Model file for the job. Use its own axes, mm. A direction names the side the tool comes from. Coordinates: 2 decimals unless noted, no trailing zeros. Write each loop counter-clockwise with the first axis right and the second up, starting at its lowest first coordinate (ties: lowest second). Pieces come first, ordered by that corner, then holes. Notation, with made-up numbers: M -2,7.25 L 23,7.25 A3 cw 23,12.25 Z; hole C 69,-2.75 d9. An arc over 180 degrees is marked long. Put each result on its own line as item: value. Start each with the question number.
Q1. Cut at B-B (z = 59.5). Write the cut outline in (x, y).
Q2. Drop flat-ended pins along their axis: pin 1 (4 mm diameter, centred on x = 11.5, z = 10, fed in from -Y); pin 2 (6 mm diameter, centred on x = 1.5, z = 39, fed in from +Y); pin 3 (1.5 mm diameter, centred on x = 10, y = -10.5, fed in from -Z); pin 4 (4 mm diameter, centred on x = -12, z = 88, fed in from -Y). Give the stop position or say it passes through.
Q3. Which spindle directions (+Z, -Z, +X, -X, +Y, -Y) get a long thin tool onto all of the face, cutting with end or side? Do faces 4 (the flat face through (-11.5, 5.9, 100)), 5 (the flat face through (0, 20, 33)), 6 (the cylindrical face through (11.923, -3.755, -32.955)). Say none if no direction does.
Q4. Cut at D-D (x = 21). Write the cut outline in (y, z), then the cut area to 3 significant figures.
Q5. Pull direction Z, two halves, no side cores. Call faces 1 (the cylindrical face through (-20, -15, 49)), 2 (the flat face through (0, 22, 70)), 3 (the flat face through (0, 0, 165)): pulls with the +Z half, pulls with the -Z half, needs draft (parallel to the pull), parting line crosses it, or undercut.
Q6. Cut at A-A (y = 0). Write the cut outline in (x, z).
Q7. Cut at C-C (z = 6). Write the cut outline in (x, y), then the cut area to 3 significant figures.
Q8. Drill centre lines: line 1 along Z through (x, y) = (19.5, -15.5); line 2 along Z through (x, y) = (-0.5, -22); line 3 along Z through (x, y) = (-11.5, -5). Where is each one in solid material? Low to high.
```python
from build123d import *

# Parameters (mm, degrees)
IZIM1_R                     = 25
Y_KSEKLIK_EKSTR_ZYON1_DEPTH = 100
IZIM2_R                     = 12.5
Y_KSEKLIK_EKSTR_ZYON2_DEPTH = 65
Y_KSEKLIK_EKSTR_ZYON3_START = 65
IZIM3_R                     = 12.5
Y_KSEKLIK_EKSTR_ZYON3_DEPTH = 65
KES_EKSTR_ZYON1_DEPTH       = 65
KES_EKSTR_ZYON1_DEPTH_BACK  = 65
KES_EKSTR_ZYON2_START       = 20
IZIM5_W                     = 40
IZIM5_H                     = 40
KES_EKSTR_ZYON2_DEPTH       = 10


with BuildPart() as part:
    # izim1 → Y_kseklik-Ekstr_zyon1 (new body)
    with BuildSketch(Plane.XY):
        Circle(IZIM1_R)
    extrude(amount=Y_KSEKLIK_EKSTR_ZYON1_DEPTH)

    # izim2 → Y_kseklik-Ekstr_zyon2 (add)
    with BuildSketch(Plane.XY.offset(100)):
        Circle(IZIM2_R)
    extrude(amount=Y_KSEKLIK_EKSTR_ZYON2_DEPTH)

    # izim3 → Y_kseklik-Ekstr_zyon3 (add)
    with BuildSketch(Plane(origin=(0, 0, 0), x_dir=(-1, 0, 0), z_dir=(0, 0, -1)).offset(Y_KSEKLIK_EKSTR_ZYON3_START)):
        with Locations(Location((0, 0, 0), (0, 0, 180))):
            Circle(IZIM3_R)
    extrude(amount=-Y_KSEKLIK_EKSTR_ZYON3_DEPTH)

    # izim4 → Kes-Ekstr_zyon1 (cut, two sides: drawn at the far end of the back side and taken through both)
    with BuildSketch(Plane(origin=(0, 0, 0), x_dir=(1, 0, 0), z_dir=(0, 1, 0)).offset(-KES_EKSTR_ZYON1_DEPTH_BACK)):
        with BuildLine():
            ThreePointArc((15, -50), (10.606601718, -39.393398282), (0, -35))
            Line((0, -35), (0, -65))
            ThreePointArc((0, -65), (10.606601718, -60.606601718), (15, -50))
        make_face()
        with BuildLine():
            Line((0, -65), (0, -35))
            ThreePointArc((0, -35), (-15, -50), (0, -65))
        make_face()
    extrude(amount=KES_EKSTR_ZYON1_DEPTH + KES_EKSTR_ZYON1_DEPTH_BACK, mode=Mode.SUBTRACT)

    # izim5 → Kes-Ekstr_zyon2 (cut)
    with BuildSketch(Plane(origin=(0, 0, 0), x_dir=(1, 0, 0), z_dir=(0, 1, 0)).offset(KES_EKSTR_ZYON2_START)):
        with Locations((0, -50)):
            Rectangle(IZIM5_W, IZIM5_H)
    extrude(amount=KES_EKSTR_ZYON2_DEPTH, mode=Mode.SUBTRACT)


solid = part.part
```
Computed values:
1. outline: M -15,20 A25 ccw -11.61,-22.14 L -11.61,20 Z; M 11.61,-22.14 A25 ccw 15,20 L 11.61,20 Z
2. pin 1: y = -23.12
2. pin 2: through
2. pin 3: z = 0
2. pin 4: y = -22.91
3. face 4: +Z
3. face 5: +X, -X, +Y
3. face 6: -Z
4. outline: M -13.56,0 L 13.56,0 L 13.56,100 L -13.56,100 Z
4. area: 2,710 mm2
5. face 1: needs draft
5. face 2: undercut
5. face 3: pulls with the +Z half
6. outline: M -25,0 L -12.5,0 L -12.5,-65 L 12.5,-65 L 12.5,0 L 25,0 L 25,100 L 12.5,100 L 12.5,165 L -12.5,165 L -12.5,100 L -25,100 Z; hole C 0,50 d30
7. outline: C 0,0 d50
7. area: 1,960 mm2
8. line 1: 0 to 100
8. line 2: 0 to 35.01, 64.99 to 100
8. line 3: 0 to 40.37, 59.63 to 100
